Autodesk Inventor part; units mm, degrees
ref_plane "YZ Plane" through (0, 0, 0) normal (1, 0, 0) x (0, 1, 0)
ref_plane "XZ Plane" through (0, 0, 0) normal (0, 1, 0) x (-1, 0, 0)
ref_plane "XY Plane" through (0, 0, 0) normal (0, 0, 1) x (1, 0, 0)
sketch "Skizze1" plane through (0, 0, 0) normal (0, 0, 1) x (1, 0, 0)
  point P0 (0, 0)
sketch "Skizze2" plane through (0, 0, 0) normal (0, 0, 1) x (1, 0, 0)
  line L0 (-15.5739, -1.2028) -> (16.4261, -1.2028)
  line L1 (16.4261, -1.2028) -> (16.4261, -10.2028)
  line L2 (16.4261, -10.2028) -> (-15.5739, -10.2028)
  line L3 (-15.5739, -10.2028) -> (-15.5739, -1.2028)
  point P0 (0, 0)
  dimension "d0" = 32
  dimension "d1" = 9
extrude "Extrusion1" add sketch "Skizze2" along normal blind 10.5
sketch "Skizze3" plane through (16.4261, -10.2028, 0) normal (1, 0, 0) x (0, 0, -1)
  point P0 (0, 10.2028)
sketch "Skizze4" plane through (-15.5739, -1.2028, 0) normal (0, 1, 0) x (1, 0, 0)
  line L0 (0, 0) -> (0, -10.5)
  line L1 (0, 0) -> (32, 0)
  point P0 (15.5739, 0)
  point P1 (16, -3.75)
  point P2 (7.496, -3.75)
  point P3 (24.504, -3.75)
  dimension "d4" = 8.504
  dimension "d5" = 8.504
  dimension "d6" = 16
  dimension "d14" = 3.75
  dimension "d15" = 3.75
hole "Bohrung1" at (-8.0779, -1.2028, 3.75) at (8.9301, -1.2028, 3.75) at (0.4261, -1.2028, 3.75) direction (0, -1, 0) diameter 6.15 end through all
sketch "Skizze5" plane through (0, 0, 0) normal (0, 0, -1) x (-1, 0, 0)
  point P0 (0, 0)
sketch "Skizze6" plane through (0, 0, 0) normal (0, 0, -1) x (-1, 0, 0)
  line L0 (-4.8511, -7.7528) -> (3.9989, -7.7528)
  line L1 (3.9989, -7.7528) -> (3.9989, -3.6528)
  line L2 (3.9989, -3.6528) -> (-4.8511, -3.6528)
  line L3 (-4.8511, -3.6528) -> (-4.8511, -7.7528)
  line L4 (-16.4261, -10.2028) -> (15.5739, -10.2028)
  line L5 (15.5739, -10.2028) -> (15.5739, -1.2028)
  point P0 (0, 0)
  dimension "d16" = 8.85
  dimension "d17" = 4.1
  dimension "d18" = 2.45
  dimension "d19" = 11.575
extrude "Extrusion2" cut sketch "Skizze6" against normal blind 9.3
sketch "Skizze7" plane through (-15.5739, -10.2028, 0) normal (0, -1, 0) x (1, 0, 0)
  point P0 (15.5739, 0)
sketch "Skizze8" plane through (0, 0, 0) normal (0, 0, -1) x (-1, 0, 0)
  point P0 (0, 0)
sketch "Skizze9" plane through (-15.5739, -10.2028, 0) normal (0, -1, 0) x (1, 0, 0)
  line L0 (0, 0) -> (32, 0)
  line L1 (4.9045, 0) -> (9.9045, 0)
  line L2 (9.9045, 0) -> (9.9045, 1.2)
  line L3 (9.9045, 1.2) -> (4.9045, 1.2)
  line L4 (4.9045, 1.2) -> (4.9045, 0)
  point P0 (15.5739, 0)
  dimension "d22" = 1.2
  dimension "d23" = 5
extrude "Extrusion3" add sketch "Skizze9" along normal blind 15
sketch "Skizze10" plane through (0, 0, 0) normal (0, 0, -1) x (-1, 0, 0)
  line L0 (5.6694, -25.2028) -> (10.6694, -25.2028)
  line L1 (15.5739, -1.2028) -> (-16.4261, -1.2028)
  line L2 (10.6694, -25.2028) -> (5.6694, -25.2028)
  line L3 (5.6694, -25.2028) -> (5.6694, -1.2028)
  line L4 (5.6694, -1.2028) -> (10.6694, -1.2028)
  line L5 (10.6694, -1.2028) -> (10.6694, -25.2028)
  point P0 (0, 0)
  dimension "d26" = 5
extrude "Extrusion4" add sketch "Skizze10" along normal blind 5
sketch "Skizze11" plane through (-15.5739, -25.2028, 0) normal (0, -1, 0) x (1, 0, 0)
  line L0 (4.9045, -5) -> (9.9045, -5)
  line L1 (6.7795, -5) -> (8.0295, -5)
  line L2 (8.0295, -5) -> (8.0295, -0.9525)
  line L3 (8.0295, -0.9525) -> (6.7795, -0.9525)
  line L4 (6.7795, -0.9525) -> (6.7795, -5)
  line L5 (9.9045, 1.2) -> (9.9045, -5)
  point P0 (15.5739, 0)
  dimension "d29" = 1.25
  dimension "d30" = 1.875
  dimension "d31" = 4.0475
extrude "Extrusion5" cut sketch "Skizze11" against normal blind 22
sketch "Skizze12" plane through (-15.5739, -25.2028, 0) normal (0, -1, 0) x (1, 0, 0)
  line L0 (9.9045, 1.2) -> (9.9045, 0)
  line L1 (4.9045, 0) -> (4.9045, 1.2)
  line L2 (9.9045, 1.2) -> (4.9045, 1.2)
  line L3 (4.9045, 1.2) -> (4.9045, 0)
  line L4 (4.9045, 0) -> (9.9045, 0)
  line L5 (9.9045, 0) -> (9.9045, 1.2)
  point P0 (15.5739, 0)
extrude "Extrusion6" cut sketch "Skizze12" against normal blind 15
sketch "Skizze13" plane through (0, 0, 0) normal (0, 1, 0) x (-1, 0, 0)
  line L0 (5.6694, 0) -> (-16.4261, 0)
  line L1 (-6.5211, 0) -> (-11.5211, 0)
  line L2 (-11.5211, 0) -> (-11.5211, -5)
  line L3 (-11.5211, -5) -> (-6.5211, -5)
  line L4 (-6.5211, -5) -> (-6.5211, 0)
  line L5 (-16.4261, 0) -> (-16.4261, 10.5)
  point P0 (0, 0)
  dimension "d36" = 5
  dimension "d37" = 5
  dimension "d38" = 4.905
extrude "Extrusion7" add sketch "Skizze13" against normal blind 25.203
sketch "Skizze14" plane through (6.5211, 0, 0) normal (0, 0, 1) x (1, 0, 0)
  line L0 (5, -1.2028) -> (9.905, -1.2028)
  line L1 (0, 0) -> (0, -25.203)
  line L2 (5, -1.2028) -> (0, -1.2028)
  line L3 (0, -1.2028) -> (0, 0)
  line L4 (0, 0) -> (5, 0)
  line L5 (5, 0) -> (5, -1.2028)
  point P0 (-6.5211, 0)
extrude "Extrusion8" cut sketch "Skizze14" against normal blind 25
sketch "Skizze15" plane through (0, -25.203, 0) normal (0, -1, 0) x (1, 0, 0)
  line L0 (6.5211, -5) -> (11.5211, -5)
  line L1 (8.3961, -5) -> (9.6461, -5)
  line L2 (9.6461, -5) -> (9.6461, -0.952)
  line L3 (9.6461, -0.952) -> (8.3961, -0.952)
  line L4 (8.3961, -0.952) -> (8.3961, -5)
  line L5 (11.5211, -5) -> (11.5211, 0)
  point P0 (0, 0)
  dimension "d43" = 1.25
  dimension "d44" = 4.048
  dimension "d45" = 1.875
extrude "Extrusion9" cut sketch "Skizze15" against normal blind 22
sketch "Skizze16" plane through (-15.5739, -25.2028, 0) normal (0, -1, 0) x (1, 0, 0)
  line L0 (0, 0) -> (4.9045, 0)
  line L1 (4.9045, -5) -> (9.9045, -5)
  line L2 (4.9045, 0) -> (9.9045, 0)
  line L3 (9.9045, 0) -> (9.9045, -5)
  line L4 (9.9045, -5) -> (4.9045, -5)
  line L5 (4.9045, -5) -> (4.9045, 0)
  point P0 (15.5739, 0)
extrude "Extrusion10" cut sketch "Skizze16" against normal blind 25
properties part number "Objektträgerhalter 3a Neu"
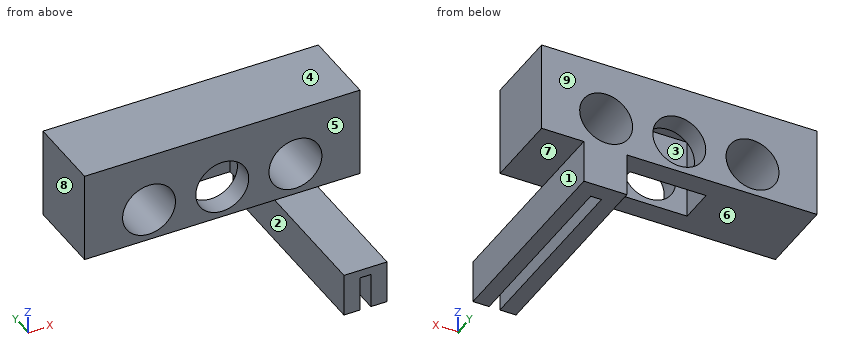
Verification items for the finished model (mm, model axes). Face numbers are marked on the shaded views. A direction names the side the tool comes from. Coordinates: 2 decimals unless noted, no trailing zeros. Order: outer loops, then holes, each group sorted by start corner. A loop starts at its lowest first (then second) coordinate and runs counter-clockwise, first axis right, second up.
1. Sectioned sample at B-B, the plane z = 3.75. Record the cut outline in (x, y).
Results found:
outline: (-15.57, -10.2) - (-11.15, -10.2) - (-11.15, -1.2) - (-15.57, -1.2) - close; (-5, -10.2) - (-2.65, -10.2) - (-2.65, -7.75) - (-4, -7.75) - (-4, -3.65) - (-2.65, -3.65) - (-2.65, -1.2) - (-5, -1.2) - close; (3.5, -10.2) - (5.86, -10.2) - (5.86, -1.2) - (3.5, -1.2) - (3.5, -3.65) - (4.85, -3.65) - (4.85, -7.75) - (3.5, -7.75) - close; (12.01, -10.2) - (16.43, -10.2) - (16.43, -1.2) - (12.01, -1.2) - close
2. Release check for a two-part mould opening along X. For the marked faces 1, 2, 3 and 4 record: +X half, -X half, draft (parallel to the pull), parting line (faces both ways), or undercut.
Results found:
face 1: +X half
face 2: -X half
face 3: undercut
face 4: draft
3. Scan lines: line 1 (X direction, y = -2.7, z = 3.75); line 2 (X direction, y = -4.25, z = 3.75); line 3 (Y direction, x = -3.5, z = 7.25). Record each from-to range of solid material in increasing order.
Results found:
line 1: x = -15.57 to -11.15, -5 to -2.65, 3.5 to 5.86, 12.01 to 16.43
line 2: x = -15.57 to -11.15, -5 to -4, 4.85 to 5.86, 12.01 to 16.43
line 3: y = -10.2 to -7.75, -3.65 to -1.2
4. Sectioned sample at A-A, the plane z = 8.75. Record the cut outline in (x, y).
Results found:
outline: (-15.57, -10.2) - (16.43, -10.2) - (16.43, -1.2) - (-15.57, -1.2) - close; hole (-4, -7.75) - (4.85, -7.75) - (4.85, -3.65) - (-4, -3.65) - close
5. Sectioned sample at D-D, the plane x = -10. Record the cut outline in (y, z), and give its area (3 significant figures).
Results found:
outline: (-10.2, 0) - (-1.2, 0) - (-1.2, 1.35) - (-10.2, 1.35) - close; (-10.2, 6.15) - (-1.2, 6.15) - (-1.2, 10.5) - (-10.2, 10.5) - close
area: 51.3 mm2
6. Go/stop test with flat-tipped pins: pin 1 Ø5 at (x, z) = (-2.5, 4) entering from -Y; pin 2 Ø4 at (y, z) = (-14, -1.5) entering from -X; pin 3 Ø5 at (x, y) = (0, -11) entering from -Z. Record where each tip stops, or that it passes through.
Results found:
pin 1: stops at y = -10.2
pin 2: stops at x = 6.52
pin 3: stops at z = 0
7. Set-up check for the marked faces 5, 6, 7, 8 and 9: record each of +Z, -Z, +X, -X, +Y, -Y from which the full face is reachable in a straight line by a thin tool's end or side.
Results found:
face 5: +Z, +X, -X, -Y
face 6: -Z, -X, +Y, -Y
face 7: -Z, +X, +Y, -Y
face 8: +Z, -Z, -X, +Y, -Y
face 9: +Z, -Z, +X, -X, +Y
8. Sectioned sample at C-C, the plane y = -6.75. Record the cut outline in (x, z) (3 decimals), and give its area (3 significant figures).
Results found:
outline: (-15.574, 0) - (-3.999, 0) - (-3.999, 9.3) - (4.851, 9.3) - (4.851, 0) - (6.521, 0) - (6.521, -5) - (8.396, -5) - (8.396, -0.952) - (9.646, -0.952) - (9.646, -5) - (11.521, -5) - (11.521, 0) - (16.426, 0) - (16.426, 10.5) - (-15.574, 10.5) - close; hole circle Ø6.15 at (-8.078, 3.75); hole circle Ø6.15 at (8.93, 3.75)
area: 214 mm2
